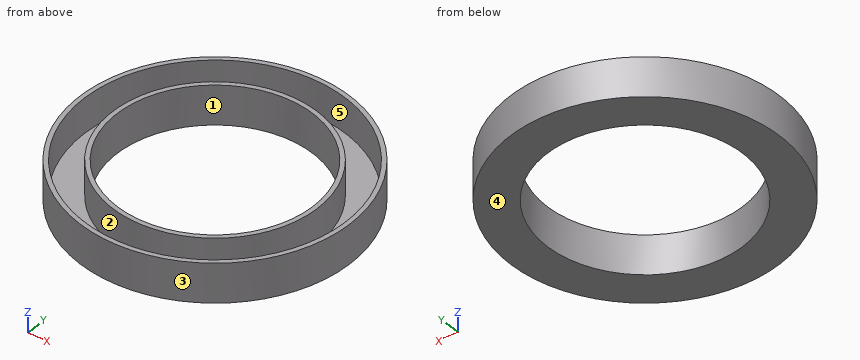
from build123d import *

# Parameters (mm, degrees)
SKETCH_1_R      = 31
SKETCH_1_R_2    = 22.5
EXTRUDE_1_DEPTH = 9
SHELL_1_T       = -1


with BuildPart() as part:
    # 草图1 → 凸台-拉伸1 (new body)
    with BuildSketch(Plane.XY):
        Circle(SKETCH_1_R)
        Circle(SKETCH_1_R_2, mode=Mode.SUBTRACT)
    extrude(amount=EXTRUDE_1_DEPTH)

    # 抽壳1
    shell_1_openings = [part.faces().sort_by_distance(p)[0] for p in [
        (-30.123187591, 0, 9),
    ]]
    offset(amount=SHELL_1_T, openings=shell_1_openings, kind=Kind.INTERSECTION)


solid = part.part
Source: CAD feature listing. Evaluate the final solid. Frame: model axes, mm. Face numbers are marked on the shaded views. A direction names the side the tool comes from. Round coordinates to 2 decimals unless told otherwise and drop trailing zeros. Loops run counter-clockwise (first coordinate to the right, second up) from the corner with the lowest first, then second, coordinate; pieces in that order, holes last.
Q1. Mould query, pull axis X, two halves, no side actions, for the marked faces 3, 4 and 5. Classes: pulls with the +X half, pulls with the -X half, needs draft (parallel to the pull), parting line crosses it, or undercut.
Q2. Access query for the marked faces 1 and 2. Directions: +Z, -Z, +X, -X, +Y, -Y. A direction counts if a zero-diameter tool reaches every point of the face in a straight line with its end or side. Return the directions, or none.
Q3. First-contact query: P1, Ø2, axis at y = 24, z = 8, coming from the -X side; P2, Ø4, axis at x = -22, z = 6.5, coming from the +Y side; P3, Ø1.5, axis at y = -20.5, z = 3, coming from the -X side. Flat tips, straight axial feed; report the tip coordinate or a pass-through.
Q4. Section B-B, the plane z = 6. Return loops of the section in (x, y), plus the area to 3 significant figures.
Q5. Ray query, line 1 (Y direction, x = 0, z = 4.5); line 2 (Y direction, x = 8.5, z = 7); line 3 (X direction, y = 4.5, z = 8). Return the intervals inside material, ascending.
Q6. Section A-A, the plane x = 0. Return loops of the section in (y, z), plus the area to 3 significant figures.
Solutions:
1. face 3: parting line crosses it
1. face 4: needs draft
1. face 5: undercut
2. face 1: +Z, -Z
2. face 2: +Z
3. P1: stops at x = -20.78
3. P2: stops at y = 23.69
3. P3: stops at x = -23.89
4. outline: circle Ø62 at (0, 0); circle Ø47 at (0, 0); hole circle Ø60 at (0, 0); hole circle Ø45 at (0, 0)
4. area: 336 mm2
5. line 1: y = -31 to -30, -23.5 to -22.5, 22.5 to 23.5, 30 to 31
5. line 2: y = -29.81 to -28.77, -21.91 to -20.83, 20.83 to 21.91, 28.77 to 29.81
5. line 3: x = -30.67 to -29.66, -23.07 to -22.05, 22.05 to 23.07, 29.66 to 30.67
6. outline: (-31, 0) - (-22.5, 0) - (-22.5, 9) - (-23.5, 9) - (-23.5, 1) - (-30, 1) - (-30, 9) - (-31, 9) - close; (22.5, 0) - (31, 0) - (31, 9) - (30, 9) - (30, 1) - (23.5, 1) - (23.5, 9) - (22.5, 9) - close
6. area: 49.0 mm2
